from build123d import *

# Parameters (mm, degrees)
AUFSATZ_LINEAR_AUSTRAGEN1_DEPTH = 330
SKIZZE2_R                       = 2.5
SCHNITT_LINEAR_AUSTRAGEN1_DEPTH = 60


with BuildPart() as part:
    # Skizze1 → Aufsatz-Linear austragen1 (new, symmetric)
    with BuildSketch(Plane.XY):
        with BuildLine():
            Line((-9, 15), (9, 15))
            ThreePointArc((9, 15), (13.242640687, 13.242640687), (15, 9))
            Line((15, 9), (15, -9))
            ThreePointArc((15, -9), (13.242640687, -13.242640687), (9, -15))
            Line((9, -15), (-9, -15))
            ThreePointArc((-9, -15), (-13.242640687, -13.242640687), (-15, -9))
            Line((-15, -9), (-15, 9))
            ThreePointArc((-15, 9), (-13.242640687, 13.242640687), (-9, 15))
        make_face()
        with BuildLine():
            Line((-13, 9), (-13, -9))
            ThreePointArc((-13, -9), (-11.828427125, -11.828427125), (-9, -13))
            Line((-9, -13), (9, -13))
            ThreePointArc((9, -13), (11.828427125, -11.828427125), (13, -9))
            Line((13, -9), (13, 9))
            ThreePointArc((13, 9), (11.828427125, 11.828427125), (9, 13))
            Line((9, 13), (-9, 13))
            ThreePointArc((-9, 13), (-11.828427125, 11.828427125), (-13, 9))
        make_face(mode=Mode.SUBTRACT)
    extrude(amount=AUFSATZ_LINEAR_AUSTRAGEN1_DEPTH, both=True)

    # Skizze2 → Schnitt-Linear austragen1 (cut)
    with BuildSketch(Plane.XZ.offset(15)):
        with Locations(Location((0, -305, 0), (0, 0, 270))):
            Circle(SKIZZE2_R)
        with Locations(Location((0, -245, 0), (0, 0, 270))):
            Circle(SKIZZE2_R)
        with Locations(Location((0, -145, 0), (0, 0, 270))):
            Circle(SKIZZE2_R)
        with Locations(Location((0, -45, 0), (0, 0, 270))):
            Circle(SKIZZE2_R)
        with Locations(Location((0, 45, 0), (0, 0, 270))):
            Circle(SKIZZE2_R)
        with Locations(Location((0, 145, 0), (0, 0, 270))):
            Circle(SKIZZE2_R)
        with Locations(Location((0, 245, 0), (0, 0, 270))):
            Circle(SKIZZE2_R)
        with Locations(Location((0, 305, 0), (0, 0, 270))):
            Circle(SKIZZE2_R)
    extrude(amount=-SCHNITT_LINEAR_AUSTRAGEN1_DEPTH, mode=Mode.SUBTRACT)


solid = part.part
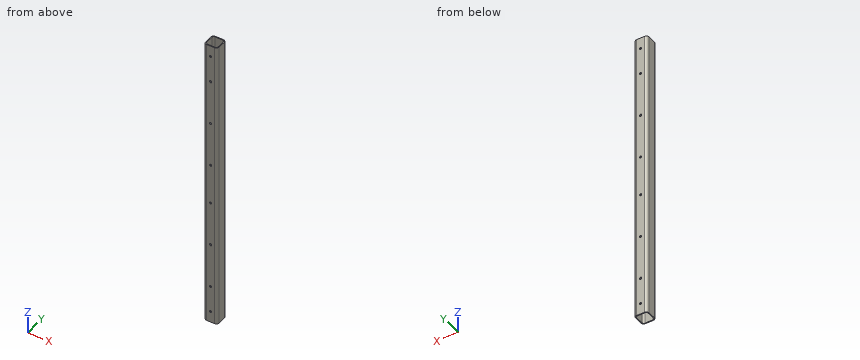
Verification items for the finished model (mm, model axes). Give positions to 0.01 mm unless a question says otherwise; leave off trailing zeros. Write each loop counter-clockwise with the first axis right and the second up, starting at its lowest first coordinate (ties: lowest second). Pieces come first, ordered by that corner, then holes. Notation, with made-up numbers: M -33.5,17.5 L -25.5,17.5 A26 ccw -25.5,36.5 Z; hole C -26,5.25 d1. An arc over 180 degrees is marked long. Put each result on its own line as item: value. Start each with the question number.
1. Section check A-A (z = 26). Record the cut outline in (x, y).
2. Scan lines: line 1 along Y through (x, z) = (-5, -224.5); line 2 along Y through (x, z) = (11.5, -119). Record each from-to range of solid material in increasing order. Write a range as [from, to].
3. Go/stop test with a flat-tipped pin: pin 1 Ø6 at (x, z) = (0, 45) entering from -Y. Record where the tip stops, or that it passes through.
4. Section check B-B (y = 4.25). Record the cut outline in (x, z), and give its area (3 significant figures).
Answer list:
1. outline: M -15,-9 A6 ccw -9,-15 L 9,-15 A6 ccw 15,-9 L 15,9 A6 ccw 9,15 L -9,15 A6 ccw -15,9 Z; hole M -13,-9 A4 ccw -9,-13 L 9,-13 A4 ccw 13,-9 L 13,9 A4 ccw 9,13 L -9,13 A4 ccw -13,9 Z
2. line 1: [-15, -13], [13, 15]
2. line 2: [-14.45, -12.12], [12.12, 14.45]
3. pin 1: y = -15
4. outline: M -15,-330 L -13,-330 L -13,330 L -15,330 Z; M 13,-330 L 15,-330 L 15,330 L 13,330 Z
4. area: 2,640 mm2
